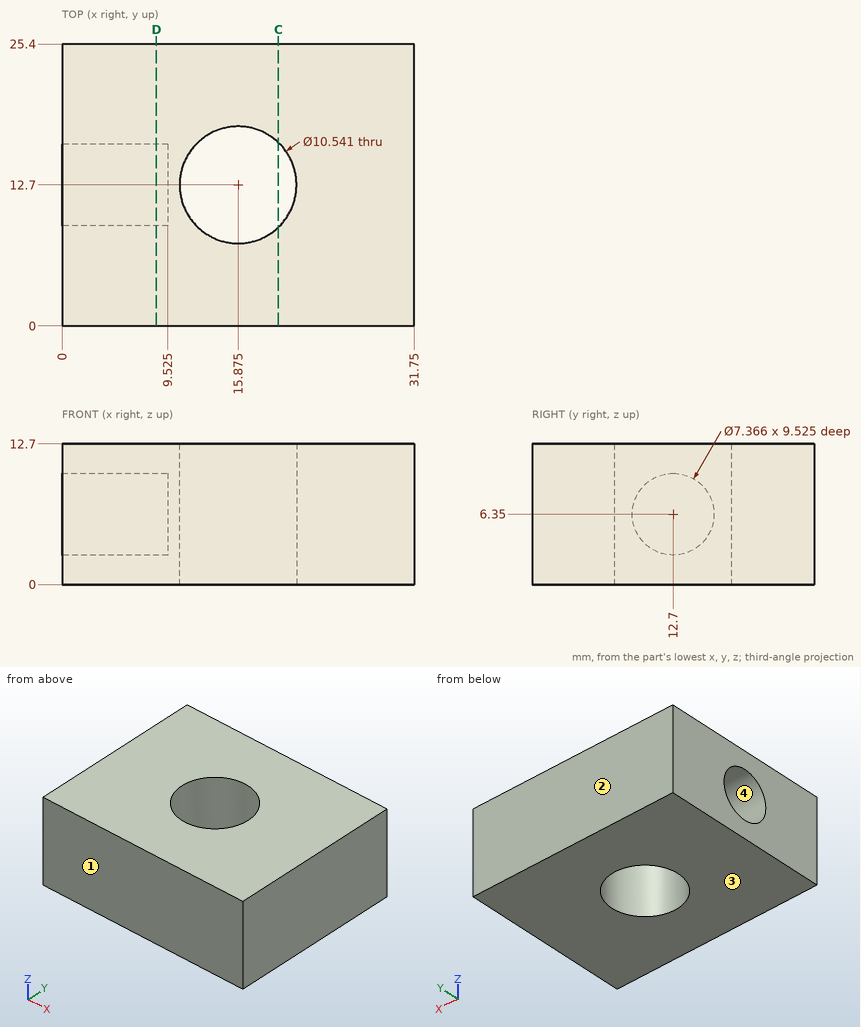
Verification items for this drawing (mm, ordinates from the low corner). Coordinates: 2 decimals unless noted, no trailing zeros. Write each loop counter-clockwise with the first axis right and the second up, starting at its lowest first coordinate (ties: lowest second). Pieces come first, ordered by that corner, then holes. Notation, with made-up numbers: M -32,-4.75 L 2,-4.75 A18 ccw 2,8.25 Z; hole C 13,71 d6. An arc over 180 degrees is marked long. Use CSV: the item, a comma, the result in double quotes.
Q1. Mould release check, pull along Y, two halves, no side actions. Record for the marked faces 1, 2, 3 and 4: pulls with the +Y half, pulls with the -Y half, needs draft (parallel to the pull), parting line crosses it, or undercut.
Computed values:
face 1,"pulls with the -Y half"
face 2,"pulls with the +Y half"
face 3,"needs draft"
face 4,"undercut"
Q2. Go/stop test with a flat-tipped pin: P1, Ø2, axis at y = 13, z = 8, coming from the -X side (3 decimals). Record where the tip stops, or that it passes through.
Computed values:
P1,"x = 9.525"
Q3. Section check C-C, the plane x = 19.5. Enter the section's corners in (y, z).
Computed values:
outline,"M 0,0 L 8.87,0 L 8.87,12.7 L 0,12.7 Z; M 16.53,0 L 25.4,0 L 25.4,12.7 L 16.53,12.7 Z"
Q4. Section check D-D, the plane x = 8.5. Enter the section's corners in (y, z).
Computed values:
outline,"M 0,0 L 25.4,0 L 25.4,12.7 L 0,12.7 Z; hole C 12.7,6.35 d7.37"
Q5. Thickness scan on line 1 along Y through (x, z) = (7, 6.35); line 2 along X through (y, z) = (12.5, 5.75) (3 decimals); line 3 along Y through (x, z) = (16, 2). Record the ranges inside material, lowest first. Write a range as [from, to].
Computed values:
line 1,"[0, 9.02], [16.38, 25.4]"
line 2,"[9.525, 10.608], [21.142, 31.75]"
line 3,"[0, 7.43], [17.97, 25.4]"
